For this review, take the finished solid that the model builds, in its own axes (mm). Give positions to 0.01 mm unless a question says otherwise; leave off trailing zeros. Order: outer loops, then holes, each group sorted by start corner. A loop starts at its lowest first (then second) coordinate and runs counter-clockwise, first axis right, second up. Notation, with made-up numbers: (-40, 30.5) - (-17, 30.5) arc R8 ccw to (-17, 38.5) - close; hole circle Ø2 at (-4.75, 60.5). An arc over 180 degrees is marked (long way). Use a Markdown table: item, result. Add a question column.
1) We need section B-B on x = 21.5. Write out the cut boundary in (y, z) (3 decimals), then the cut area to 3 significant figures.
2) We need section D-D on z = 10. Write out the cut boundary in (x, y) (3 decimals).
3) We need section C-C on y = 2.25. Write out the cut boundary in (x, z) (3 decimals), then the cut area to 3 significant figures.
4) Wall thickness on L1, parallel to X at y = 3.05, z = -9.5 (3 decimals); L2, parallel to X at y = 2.2, z = 0 (3 decimals); L3, parallel to Z at x = -23.5, y = 1.2 (3 decimals): over which ranges is each line inside the solid? List them lowest first.
5) We need section A-A on z = 0. Write out the cut boundary in (x, y) (3 decimals), then the cut area to 3 significant figures.
6) Clearance check with a flat-ended pin moving along its axis: P1, Ø2.5, axis at x = 22.22, z = 10.32, coming from the +Y side. State where the tip first meets the part, or that it passes through.
7) Mouldability with a two-part tool opening along Z and no side actions: class faces 1 (the face through (0, 2, 15.875)), 2 (the face through (28.575, 2, 0)), 3 (the face through (0.741, 1.565, -3.174)) as released by +Z, released by -Z, zero draft, split by the parting line, or undercut.
```python
from build123d import *

# Parameters (mm, degrees)
SKETCH1_W           = 57.15
SKETCH1_H           = 31.75
SKETCH1_R           = 4
BOSS_EXTRUDE1_DEPTH = 3.175
FILLET1_R           = 3.81
SKETCH2_R           = 2.032
CUT_EXTRUDE1_DEPTH  = 33.842455374


with BuildPart() as part:
    # Sketch1 → Boss-Extrude1 (new body)
    with BuildSketch(Plane(origin=(0, 0, 0), x_dir=(1, 0, 0), z_dir=(0, 1, 0))):
        Rectangle(SKETCH1_W, SKETCH1_H)
        with Locations(Location((3.175, 0, 0), (0, 0, 270))):
            Circle(SKETCH1_R, mode=Mode.SUBTRACT)
    extrude(amount=BOSS_EXTRUDE1_DEPTH)

    # Fillet1
    fillet1_edges = [part.edges().sort_by_distance(p)[0] for p in [
        (28.575, 1.5875, 15.875),
        (-28.575, 1.5875, 15.875),
        (-28.575, 1.5875, -15.875),
        (28.575, 1.5875, -15.875),
    ]]
    fillet(fillet1_edges, radius=FILLET1_R)

    # Sketch2 → Cut-Extrude1 (cut, through all)
    with BuildSketch(Plane.XZ):
        with Locations(Location((22.225, -10.31875, 0), (0, 0, 270))):
            Circle(SKETCH2_R)
        with Locations(Location((22.225, 10.31875, 0), (0, 0, 270))):
            Circle(SKETCH2_R)
        with Locations(Location((-22.225, -10.31875, 0), (0, 0, 270))):
            Circle(SKETCH2_R)
        with Locations(Location((-22.225, 10.31875, 0), (0, 0, 270))):
            Circle(SKETCH2_R)
    extrude(amount=-CUT_EXTRUDE1_DEPTH, mode=Mode.SUBTRACT)


solid = part.part
```
Checked values:
| question | item | result |
|---|---|---|
| 1 | outline | (0, -15.875) - (3.175, -15.875) - (3.175, -12.217) - (0, -12.217) - close; (0, -8.42) - (3.175, -8.42) - (3.175, 8.42) - (0, 8.42) - close; (0, 12.217) - (3.175, 12.217) - (3.175, 15.875) - (0, 15.875) - close |
| 1 | area | 76.7 mm² |
| 2 | outline | (-28.575, 0) - (-24.232, 0) - (-24.232, 3.175) - (-28.575, 3.175) - close; (-20.218, 0) - (20.218, 0) - (20.218, 3.175) - (-20.218, 3.175) - close; (24.232, 0) - (28.575, 0) - (28.575, 3.175) - (24.232, 3.175) - close |
| 3 | outline | (-28.575, -12.065) arc R3.81 ccw to (-24.765, -15.875) - (24.765, -15.875) arc R3.81 ccw to (28.575, -12.065) - (28.575, 12.065) arc R3.81 ccw to (24.765, 15.875) - (-24.765, 15.875) arc R3.81 ccw to (-28.575, 12.065) - close; hole circle Ø4.064 at (-22.225, -10.319); hole circle Ø4.064 at (-22.225, 10.319); hole circle Ø8 at (3.175, 0); hole circle Ø4.064 at (22.225, -10.319); hole circle Ø4.064 at (22.225, 10.319) |
| 3 | area | 1,700 mm² |
| 4 | L1 | -28.575 to -24.085, -20.365 to 20.365, 24.085 to 28.575 |
| 4 | L2 | -28.575 to -0.825, 7.175 to 28.575 |
| 4 | L3 | -15.875 to -11.901, -8.737 to 8.737, 11.901 to 15.875 |
| 5 | outline | (-28.575, 0) - (-0.825, 0) - (-0.825, 3.175) - (-28.575, 3.175) - close; (7.175, 0) - (28.575, 0) - (28.575, 3.175) - (7.175, 3.175) - close |
| 5 | area | 156 mm² |
| 6 | P1 | through |
| 7 | face 1 | released by +Z |
| 7 | face 2 | zero draft |
| 7 | face 3 | undercut |
